```python
from build123d import *

# Parameters (mm, degrees)
F1_DEPTH      = 400
F2_W          = 150
F2_H          = 5
F2_W_2        = 75
F3_DEPTH      = 645
F4_W          = 2.5
F4_H          = 50
F5_DEPTH      = 21
F6_R          = 2
F8_DEPTH      = 143
F8_DEPTH_BACK = 143
F9_R          = 2


with BuildPart() as f1:
    # F0 (on Front) → F1 (new body)
    with BuildSketch(Plane.XZ):
        with BuildLine():
            ThreePointArc((150, 148), (148.6819805153, 151.1819805153), (145.5, 152.5))
            Line((145.5, 152.5), (0, 152.5))
            Line((0, 152.5), (-145.5, 152.5))
            ThreePointArc((-145.5, 152.5), (-148.6819805153, 151.1819805153), (-150, 148))
            Line((-150, 148), (-150, 100.5))
            ThreePointArc((-150, 100.5), (-149.7286167935, 98.960909355), (-148.947199994, 97.6074557564))
            Line((-148.947199994, 97.6074557564), (-148.5848888922, 97.1756701992))
            ThreePointArc((-148.5848888922, 97.1756701992), (-148.150768448, 96.4237515333), (-148, 95.5687011749))
            Line((-148, 95.5687011749), (-148, -152.5))
            Line((-148, -152.5), (-146, -152.5))
            Line((-146, -152.5), (-146, 95.5687011749))
            ThreePointArc((-146, 95.5687011749), (-146.2713832065, 97.1077918199), (-147.052800006, 98.4612454185))
            Line((-147.052800006, 98.4612454185), (-147.4151111078, 98.8930309758))
            ThreePointArc((-147.4151111078, 98.8930309758), (-147.849231552, 99.6449496417), (-148, 100.5))
            Line((-148, 100.5), (-148, 148))
            ThreePointArc((-148, 148), (-147.267766953, 149.767766953), (-145.5, 150.5))
            Line((-145.5, 150.5), (0, 150.5))
            Line((0, 150.5), (145.5, 150.5))
            ThreePointArc((145.5, 150.5), (147.267766953, 149.767766953), (148, 148))
            Line((148, 148), (148, 100.5))
            ThreePointArc((148, 100.5), (147.849231552, 99.6449496417), (147.4151111078, 98.8930309758))
            Line((147.4151111078, 98.8930309758), (147.052800006, 98.4612454185))
            ThreePointArc((147.052800006, 98.4612454185), (146.2713832065, 97.1077918199), (146, 95.5687011749))
            Line((146, 95.5687011749), (146, -152.5))
            Line((146, -152.5), (148, -152.5))
            Line((148, -152.5), (148, 95.5687011749))
            ThreePointArc((148, 95.5687011749), (148.150768448, 96.4237515333), (148.5848888922, 97.1756701992))
            Line((148.5848888922, 97.1756701992), (148.947199994, 97.6074557564))
            ThreePointArc((148.947199994, 97.6074557564), (149.7286167935, 98.960909355), (150, 100.5))
            Line((150, 100.5), (150, 148))
        make_face()
    extrude(amount=F1_DEPTH)

    # F2 (on face) → F3 (cut)
    with BuildSketch(Plane.YZ.offset(148)):
        with Locations((-200, -150)):
            Rectangle(F2_W, F2_H)
        with Locations((-37.5, -150)):
            Rectangle(F2_W_2, F2_H)
        with Locations((-362.5, -150)):
            Rectangle(F2_W_2, F2_H)
    extrude(amount=-F3_DEPTH, mode=Mode.SUBTRACT)

    # F4 (on face) → F5 (cut)
    with BuildSketch(Plane.XY.offset(152.5)):
        with Locations((146.75, -100)):
            Rectangle(F4_W, F4_H)
        with Locations((146.75, -300)):
            Rectangle(F4_W, F4_H)
        with Locations((-146.75, -100)):
            Rectangle(F4_W, F4_H)
        with Locations((-146.75, -300)):
            Rectangle(F4_W, F4_H)
    extrude(amount=-F5_DEPTH, mode=Mode.SUBTRACT)

    # F6
    f6_edges = [f1.edges().sort_by_distance(p)[0] for p in [
        (147, -125, -147.5),
        (147, -325, -147.5),
        (-147, -325, -147.5),
        (-147, -125, -147.5),
        (147, -75, -147.5),
        (147, -275, -147.5),
        (-147, -275, -147.5),
        (-147, -75, -147.5),
        (147, -325, -152.5),
        (147, -125, -152.5),
        (-147, -325, -152.5),
        (-147, -125, -152.5),
        (147, -275, -152.5),
        (147, -75, -152.5),
        (-147, -275, -152.5),
        (-147, -75, -152.5),
    ]]
    fillet(f6_edges, radius=F6_R)

    # F7 (on Right) → F8 (join, two sides)
    with BuildSketch(Plane.YZ) as f8_sk:
        with BuildLine():
            Line((1, 152.5), (0, 152.5))
            Line((0, 152.5), (0, 150.5))
            Line((0, 150.5), (1, 150.5))
            ThreePointArc((1, 150.5), (2.767766953, 149.767766953), (3.5, 148))
            Line((3.5, 148), (3.5, 147))
            Line((3.5, 147), (5.5, 147))
            Line((5.5, 147), (5.5, 148))
            ThreePointArc((5.5, 148), (4.1819805153, 151.1819805153), (1, 152.5))
        make_face()
    extrude(amount=F8_DEPTH)
    extrude(f8_sk.sketch, amount=-F8_DEPTH_BACK)

    # F9 (call 1 of 4: OpenCascade refuses the feature's edges together)
    f9_edges = [f1.edges().sort_by_distance(p)[0] for p in [
        (143, 0, 151.5),
    ]]
    fillet(f9_edges, radius=F9_R)

    # F9#2 (call 2 of 4)
    f9_2_edges = [f1.edges().sort_by_distance(p)[0] for p in [
        (-143, 0, 151.5),
    ]]
    fillet(f9_2_edges, radius=F9_R)

    # F9#3 (call 3 of 4)
    f9_3_edges = [f1.edges().sort_by_distance(p)[0] for p in [
        (-143, 4.5, 147),
    ]]
    fillet(f9_3_edges, radius=F9_R)

    # F9#4 (call 4 of 4)
    f9_4_edges = [f1.edges().sort_by_distance(p)[0] for p in [
        (143, 4.5, 147),
    ]]
    fillet(f9_4_edges, radius=F9_R)


solid = f1.part
```
Verification items for the finished model (mm, model axes). A direction names the side the tool comes from. Give positions to 0.01 mm unless a question says otherwise; leave off trailing zeros. Order: outer loops, then holes, each group sorted by start corner. A loop starts at its lowest first (then second) coordinate and runs counter-clockwise, first axis right, second up. Notation, with made-up numbers: (25.25, -17.5) - (76.25, -17.5) arc R34 cw to (76.25, 21.5) - close; hole circle Ø9 at (85, 85.5). An arc over 180 degrees is marked (long way). Answer as CSV lines item,"result". Start each with the question number.
Item 1: Mould release check, pull along Z, two halves, no side actions. Record for faces 4 (the face through (148, -203, 126)), 5 (the face through (150, -197, 124)), 6 (the face through (2, -197, 152.5)), 7 (the face through (2, -202, 150.5)): released by +Z, released by -Z, zero draft, split by the parting line, or undercut.
Item 2: Material ranges on L1, parallel to X at y = -143.5, z = -37; L2, parallel to X at y = -30, z = 121.5; L3, parallel to Z at x = 120, y = -193.5, recorded low to high.
Item 3: Section check C-C, the plane x = -61. Record the boundary of the cut face in (y, z).
Item 4: Section check B-B, the plane z = -82.5. Record the boundary of the cut face in (x, y), plus the area to 3 significant figures.
Item 5: Section check D-D, the plane y = -244.5. Record the boundary of the cut face in (x, z).
Item 6: Section check A-A, the plane y = -113.5. Record the boundary of the cut face in (x, z).
Item 7: Access from +Z, -Z, +X, -X, +Y, -Y to the whole of each face (thin tool, end or side, straight path). Record for faces 1 (the face through (-148, -197, -27)), 2 (the face through (146, -197, -27)), 3 (the face through (148, -197, -30)).
Item 8: Gauge pin test, flat ends, axial feed: pin 1 (0.5 mm diameter, centred on x = 146.5, z = -150, fed in from -Y); pin 2 (1 mm diameter, centred on y = 4, z = 151, fed in from +X); pin 3 (1.6 mm diameter, centred on x = -147, y = -207, fed in from -Z). Record the tip position at first contact, or that the pin passes through.
Filled in:
1,face 4,"undercut"
1,face 5,"zero draft"
1,face 6,"released by +Z"
1,face 7,"released by -Z"
2,L1,"-148 to -146, 146 to 148"
2,L2,"-150 to -148, 148 to 150"
2,L3,"150.5 to 152.5"
3,outline,"(-400, 150.5) - (1, 150.5) arc R2.5 cw to (3.5, 148) - (3.5, 147) - (5.5, 147) - (5.5, 148) arc R4.5 ccw to (1, 152.5) - (-400, 152.5) - close"
4,outline,"(-148, -400) - (-146, -400) - (-146, 0) - (-148, 0) - close; (146, -400) - (148, -400) - (148, 0) - (146, 0) - close"
4,area,"1,600 mm^2"
5,outline,"(-150, 100.5) arc R4.5 ccw to (-148.95, 97.61) - (-148.58, 97.18) arc R2.5 cw to (-148, 95.57) - (-148, -147.5) - (-146, -147.5) - (-146, 95.57) arc R4.5 ccw to (-147.05, 98.46) - (-147.42, 98.89) arc R2.5 cw to (-148, 100.5) - (-148, 148) arc R2.5 cw to (-145.5, 150.5) - (145.5, 150.5) arc R2.5 cw to (148, 148) - (148, 100.5) arc R2.5 cw to (147.42, 98.89) - (147.05, 98.46) arc R4.5 ccw to (146, 95.57) - (146, -147.5) - (148, -147.5) - (148, 95.57) arc R2.5 cw to (148.58, 97.18) - (148.95, 97.61) arc R4.5 ccw to (150, 100.5) - (150, 148) arc R4.5 ccw to (145.5, 152.5) - (-145.5, 152.5) arc R4.5 ccw to (-150, 148) - close"
6,outline,"(-150, 100.5) arc R4.5 ccw to (-148.95, 97.61) - (-148.58, 97.18) arc R2.5 cw to (-148, 95.57) - (-148, -152.5) - (-146, -152.5) - (-146, 95.57) arc R4.5 ccw to (-147.05, 98.46) - (-147.42, 98.89) arc R2.5 cw to (-148, 100.5) - (-148, 151.74) arc R4.5 ccw to (-150, 148) - close; (-145.5, 150.5) - (145.5, 150.5) - (145.5, 152.5) - (-145.5, 152.5) - close; (146, -152.5) - (148, -152.5) - (148, 95.57) arc R2.5 cw to (148.58, 97.18) - (148.95, 97.61) arc R4.5 ccw to (150, 100.5) - (150, 148) arc R4.5 ccw to (148, 151.74) - (148, 100.5) arc R2.5 cw to (147.42, 98.89) - (147.05, 98.46) arc R4.5 ccw to (146, 95.57) - close"
7,face 1,"-Z, -X, +Y, -Y"
7,face 2,"-Z, +Y, -Y"
7,face 3,"-Z, +X, +Y, -Y"
8,pin 1,"y = -325"
8,pin 2,"x = 143"
8,pin 3,"z = -147.5"
